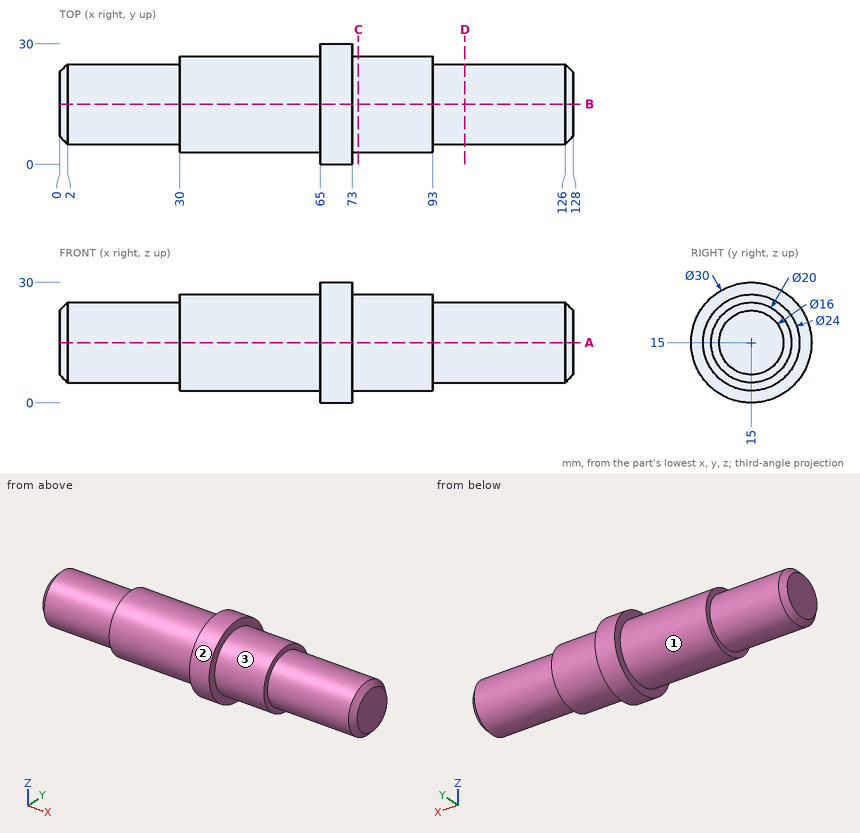
The drawing under review shows one solid part. Ordinate dimensions are in mm from its lowest x, y, z. A direction names the side the tool comes from. Round coordinates to 2 decimals unless told otherwise and drop trailing zeros. Order: outer loops, then holes, each group sorted by start corner. A loop starts at its lowest first (then second) coordinate and runs counter-clockwise, first axis right, second up. Notation, with made-up numbers: (-25, 41.5) - (5, 41.5) arc R16 cw to (5, 55.5) - close; hole circle Ø9 at (4, 45.25). An arc over 180 degrees is marked (long way). Return JSON: item names as keys, results as strings.
Q1. Machinability: for the marked faces 1, 2 and 3, which of the approach directions +Z, -Z, +X, -X, +Y, -Y give a long, thin tool a straight path to every point of the face, cutting with its end or side? Answer none if there is none.
Computed values:
{"face 1": "-X", "face 2": "+X, -X", "face 3": "+X"}
Q2. Consider section D-D on x = 101. Write out the cut boundary in (y, z).
Computed values:
{"outline": "circle Ø20 at (15, 15)"}
Q3. Consider section A-A on z = 15. Write out the cut boundary in (x, y), plus the area to 3 significant figures.
Computed values:
{"outline": "(0, 7) - (2, 5) - (30, 5) - (30, 3) - (65, 3) - (65, 0) - (73, 0) - (73, 3) - (93, 3) - (93, 5) - (126, 5) - (128, 7) - (128, 23) - (126, 25) - (93, 25) - (93, 27) - (73, 27) - (73, 30) - (65, 30) - (65, 27) - (30, 27) - (30, 25) - (2, 25) - (0, 23) - close", "area": "2,850 mm2"}
Q4. For pin 1 Ø12 at (x, z) = (33.5, 17.5) entering from -Y; pin 2 Ø4 at (x, z) = (113.5, 15.5) entering from +Y; pin 3 Ø1 at (y, z) = (4, 15) entering from +X; pin 4 Ø7 at (y, z) = (21, 14.5) entering from -X, all flat-tipped, find the tip position at first contact; note any pin that passes through.
Computed values:
{"pin 1": "stops at y = 3", "pin 2": "stops at y = 25", "pin 3": "stops at x = 93", "pin 4": "stops at x = 0"}
Q5. Consider section C-C on x = 74.5. Write out the cut boundary in (y, z).
Computed values:
{"outline": "circle Ø24 at (15, 15)"}
Q6. Wall thickness on L1, parallel to X at y = 26, z = 11.25; L2, parallel to X at y = 27.75, z = 9.75; L3, parallel to Z at x = 70.5, y = 6: over which ranges is each line inside the solid? List them lowest first. Write a range as [from, to].
Computed values:
{"L1": "x = [30, 93]", "L2": "x = [65, 73]", "L3": "z = [3, 27]"}
